The model under review builds one solid part; all positions refer to its coordinate system, in mm. A direction names the side the tool comes from. Coordinates: 2 decimals unless noted, no trailing zeros. Loops run counter-clockwise (first coordinate to the right, second up) from the corner with the lowest first, then second, coordinate; pieces in that order, holes last. Notation, with made-up numbers: M 31.25,87 L 58.25,87 A18 ccw 58.25,110 Z; hole C -31,-33.5 d3. An arc over 180 degrees is marked long. Use one line per item in the form item = value.
Autodesk Inventor part; units mm, degrees
ref_plane "YZ Plane" through (0, 0, 0) normal (1, 0, 0) x (0, 1, 0)
ref_plane "XZ Plane" through (0, 0, 0) normal (0, 1, 0) x (-1, 0, 0)
ref_plane "XY Plane" through (0, 0, 0) normal (0, 0, 1) x (1, 0, 0)
sketch "Sketch1" plane through (0, 0, 0) normal (0, 1, 0) x (-1, 0, 0)
  line L0 (0, 0) -> (0, 3.7)
  line L1 (0, 3.7) -> (1.1, 3.7)
  line L2 (1.1, 8.7) -> (0, 8.7)
  line L3 (0, 8.7) -> (0, 9.9)
  line L4 (0, 9.9) -> (4, 9.9)
  line L5 (4, 9.9) -> (4, 8.7)
  line L6 (4, 8.7) -> (2.6, 8.7)
  line L7 (2.6, 8.7) -> (2.6, 3.7)
  line L8 (2.6, 3.7) -> (1.8, 3.7)
  line L9 (1.8, 3.7) -> (1.8, 0)
  line L10 (1.8, 0) -> (0, 0)
  line L11 (1.1, 3.7) -> (1.1, 8.7)
  dimension "d0" = 3.7
  dimension "d1" = 1.8
  dimension "d2" = 1.1
  dimension "d3" = 1.2
  dimension "d4" = 1.5
  dimension "d5" = 5
  dimension "d6" = 4
extrude "Extrusion1" add sketch "Sketch1" along normal blind 10
sketch "Sketch2" plane through (0, 0, 3.7) normal (1, 0, 0) x (0, 0, -1)
  line L0 (0, 0) -> (0, 10)
  line L1 (0, 0) -> (4, 0)
  line L2 (4, 0) -> (4, 2)
  line L3 (4, 2) -> (0, 2)
  line L4 (0, 2) -> (0, 0)
  line L5 (0, 5) -> (3.7, 5) construction
  line L6 (0, 10) -> (4, 10)
  line L7 (4, 10) -> (4, 8)
  line L8 (4, 8) -> (0, 8)
  line L9 (0, 8) -> (0, 10)
  point P0 (3.7, 0)
  dimension "d9" = 6
  dimension "d10" = 4
extrude "Extrusion2" cut sketch "Sketch2" against normal up to next
sketch "Sketch3" plane through (0, 8, 0) normal (0, 0, -1) x (-1, 0, 0)
  circle A0 centre (0.9, -1.12) radius 0.3
  circle A1 centre (0.9, -2.38) radius 0.3
  circle A2 centre (0.9, -3.64) radius 0.3
  circle A3 centre (0.9, -4.9) radius 0.3
  line L0 (0, -6) -> (1.8, -6)
  line L1 (0, -6) -> (0, 0)
  line L2 (0.9, -4.9) -> (0.9, -1.12) construction
  point P0 (0, -8)
  dimension "d13" = 0.6
  dimension "d14" = 1.26
  dimension "d15" = 1.26
  dimension "d16" = 1.26
  dimension "d17" = 1.1
  dimension "d18" = 0.9
extrude "Extrusion3" cut sketch "Sketch3" against normal blind 3
sketch "Sketch4" plane through (-4, 0, 8.7) normal (-1, 0, 0) x (0, 0, 1)
  circle A0 centre (0.6, 8.2) radius 0.3
  circle A1 centre (0.6, 6.6) radius 0.3
  circle A2 centre (0.6, 5) radius 0.3
  circle A3 centre (0.6, 3.4) radius 0.3
  circle A4 centre (0.6, 1.8) radius 0.3
  line L0 (1.2, 0) -> (0, 0)
  line L1 (0.6, 0) -> (0.6, 9.9899) construction
  point P0 (-8.7, 0)
  dimension "d21" = 0.6
  dimension "d22" = 1.6
  dimension "d23" = 1.6
  dimension "d24" = 1.6
  dimension "d25" = 1.6
  dimension "d26" = 1.8
extrude "Extrusion4" add sketch "Sketch4" along normal blind 4.6
properties part number "humidity_sensor_mount"
1. Insertion check: P1, Ø2, axis at x = -3.5, y = 8.5, coming from the -Z side; P2, Ø1.1, axis at y = 4, z = 2, coming from the -X side; P3, Ø1.4, axis at x = -1, z = 2, coming from the -Y side. Each pin has a flat end and moves straight along its axis. Give the tip position at first contact, or say it passes through.
Response values:
P1 = 3.7
P2 = -1.8
P3 = 2
2. Machinability: for faces 4 (the face through (-1.8, 5, 2)), 5 (the face through (-1, 2, 2)), 6 (the face through (-0.5, 5, 3.7)), 7 (the face through (-2, 0, 8)), which of the approach directions +Z, -Z, +X, -X, +Y, -Y give a long, thin tool a straight path to every point of the face, cutting with its end or side? Answer none if there is none.
Response values:
face_4 = -Z, -X, +Y, -Y
face_5 = -Z, +X, -X, -Y
face_6 = +X, +Y, -Y
face_7 = +Z, -Z, +X, -X, -Y
3. Add section C-C (x = -6.25). State the section outline as (y, z) points.
Response values:
outline = C 1.8,9.3 d0.6; C 3.4,9.3 d0.6; C 5,9.3 d0.6; C 6.6,9.3 d0.6; C 8.2,9.3 d0.6
4. Add section D-D (z = 9.3). State the section outline as (x, y) points.
Response values:
outline = M -8.6,1.5 L -4,1.5 L -4,0 L 0,0 L 0,10 L -4,10 L -4,8.5 L -8.6,8.5 L -8.6,7.9 L -4,7.9 L -4,6.9 L -8.6,6.9 L -8.6,6.3 L -4,6.3 L -4,5.3 L -8.6,5.3 L -8.6,4.7 L -4,4.7 L -4,3.7 L -8.6,3.7 L -8.6,3.1 L -4,3.1 L -4,2.1 L -8.6,2.1 Z
5. Add section B-B (y = 5). State the section outline as (x, z) points.
Response values:
outline = M -8.6,9 L -4,9 L -4,8.7 L -2.6,8.7 L -2.6,3.7 L -1.8,3.7 L -1.8,0 L 0,0 L 0,3.7 L -1.1,3.7 L -1.1,8.7 L 0,8.7 L 0,9.9 L -4,9.9 L -4,9.6 L -8.6,9.6 Z
6. The part is to be moulded in two halves that separate along Z. For faces 1 (the face through (-1.1, 5, 6)), 2 (the face through (-2, 5, 9.9)), 3 (the face through (-1, 8, 2)), say which applies: pulls with the +Z half, pulls with the -Z half, needs draft (parallel to the pull), parting line crosses it, or undercut.
Response values:
face_1 = undercut
face_2 = pulls with the +Z half
face_3 = needs draft
7. Wall thickness on line 1 along Y through (x, z) = (-6, 9.25); line 2 along Y through (x, z) = (-0.9, 2.2); line 3 along Z through (x, y) = (-2.75, 6.5): over which ranges is each line inside the solid? List them lowest first. Write a range as from..to.
Response values:
line_1 = 1.5..2.1, 3.1..3.7, 4.7..5.3, 6.3..6.9, 7.9..8.5
line_2 = 2..2.8, 3.4..4.06, 4.66..5.32, 5.92..6.58, 7.18..8
line_3 = 8.7..9.9
8. Add section A-A (z = 2.5). State the section outline as (x, y) points.
Response values:
outline = M -1.8,2 L 0,2 L 0,8 L -1.8,8 Z; hole C -0.9,3.1 d0.6; hole C -0.9,4.36 d0.6; hole C -0.9,5.62 d0.6; hole C -0.9,6.88 d0.6
